Build history of the part. All positions in model axes, mm. A direction names the side the tool comes from. Round coordinates to 2 decimals unless told otherwise and drop trailing zeros. Write each loop counter-clockwise with the first axis right and the second up, starting at its lowest first coordinate (ties: lowest second). Pieces come first, ordered by that corner, then holes. Notation, with made-up numbers: M 27.5,35 L 46.5,35 A17 cw 46.5,53 Z; hole C 54.25,-22.75 d10. An arc over 180 degrees is marked long. Write item = value, one per line. Start each with the question number.
Q1. Band-saw the part on B-B on y = -1.2. State how many separate pieces and enclosed holes the cut face has, plus the area to 3 significant figures.
Q2. Band-saw the part on D-D on x = 44. Write the cut outline in (y, z).
Q3. Band-saw the part on A-A on x = 35. Write the cut outline in (y, z), plus the area to 3 significant figures.
Q4. Band-saw the part on C-C on x = 53.7. Write the cut outline in (y, z), plus the area to 3 significant figures.
Q5. Drop a flat-ended pin along its axis: P1, Ø5, axis at x = 28.3, z = -55.43, coming from the -Y side. Give the stop position or say it passes through.
Q6. Pull direction Z, two halves, no side cores. Call faces 3 (the cylindrical face through (50.53, -2.35, -55.57)), 4 (the flat face through (41, -2, -65)), 5 (the cylindrical face through (25.78, -2.348, -53.494)), 6 (the flat face through (36.412, -2, -2)): released by +Z, released by -Z, zero draft, split by the parting line, or undercut.
Q7. Probe L1, parallel to Z at x = 28.3, y = -3.3; L2, parallel to X at y = -0.5, z = -56.5; L3, parallel to Z at x = 47, y = -3.35. List the from-to ranges inside material, lowest first.
Q8. Tool access for faces 1 (the flat face through (16, -2, -34)), 2 (the flat face through (42.412, -2, -2)): list every direction of +Z, -Z, +X, -X, +Y, -Y with a clear straight run to the whole face (end or side of a thin tool).
```python
from build123d import *

# Parameters (mm, degrees)
SKETCH1_R           = 0.7
SKETCH1_R_2         = 3.175
BOSS_EXTRUDE1_DEPTH = 4.7625


with BuildPart() as part:
    # Sketch1 → Boss-Extrude1 (new body)
    with BuildSketch(Plane(origin=(0, 0, 0), x_dir=(1, 0, 0), z_dir=(0, 1, 0))):
        with BuildLine():
            Line((16, 1.185131266), (36.4125, 1.185131266))
            Line((36.4125, 1.185131266), (36.4125, 2.47623548))
            ThreePointArc((36.4125, 2.47623548), (38, 4.06373548), (39.5875, 2.47623548))
            Line((39.5875, 2.47623548), (39.5875, 1.185131266))
            Line((39.5875, 1.185131266), (42.4125, 1.185131266))
            Line((42.4125, 1.185131266), (42.4125, 2.47623548))
            ThreePointArc((42.4125, 2.47623548), (44, 4.06373548), (45.5875, 2.47623548))
            Line((45.5875, 2.47623548), (45.5875, 1.185131266))
            Line((45.5875, 1.185131266), (66, 1.185131266))
            Line((66, 1.185131266), (66, 65))
            Line((66, 65), (16, 65))
            Line((16, 65), (16, 1.185131266))
        make_face()
        with Locations((35, 4.197327459)):
            Circle(SKETCH1_R, mode=Mode.SUBTRACT)
        with Locations((53.7, 55.426122104)):
            Circle(SKETCH1_R_2, mode=Mode.SUBTRACT)
        with Locations((28.3, 55.426122104)):
            Circle(SKETCH1_R_2, mode=Mode.SUBTRACT)
        with Locations((47, 4.197327459)):
            Circle(SKETCH1_R, mode=Mode.SUBTRACT)
    extrude(amount=-BOSS_EXTRUDE1_DEPTH)


solid = part.part
```
Conclusion:
q1.separate_pieces = 1
q1.enclosed_holes = 4
q1.area = 3,110 mm^2
q2.outline = M -4.76,-65 L 0,-65 L 0,-4.06 L -4.76,-4.06 Z
q3.outline = M -4.76,-65 L 0,-65 L 0,-4.9 L -4.76,-4.9 Z; M -4.76,-3.5 L 0,-3.5 L 0,-1.19 L -4.76,-1.19 Z
q3.area = 297 mm^2
q4.outline = M -4.76,-65 L 0,-65 L 0,-58.6 L -4.76,-58.6 Z; M -4.76,-52.25 L 0,-52.25 L 0,-1.19 L -4.76,-1.19 Z
q4.area = 274 mm^2
q5.P1 = through
q6.face_3 = undercut
q6.face_4 = released by -Z
q6.face_5 = undercut
q6.face_6 = zero draft
q7.L1 = -65 to -58.6, -52.25 to -1.19
q7.L2 = 16 to 25.31, 31.29 to 50.71, 56.69 to 66
q7.L3 = -65 to -4.9, -3.5 to -1.19
q8.face_1 = +Z, -Z, -X, +Y, -Y
q8.face_2 = +Z, +Y, -Y
